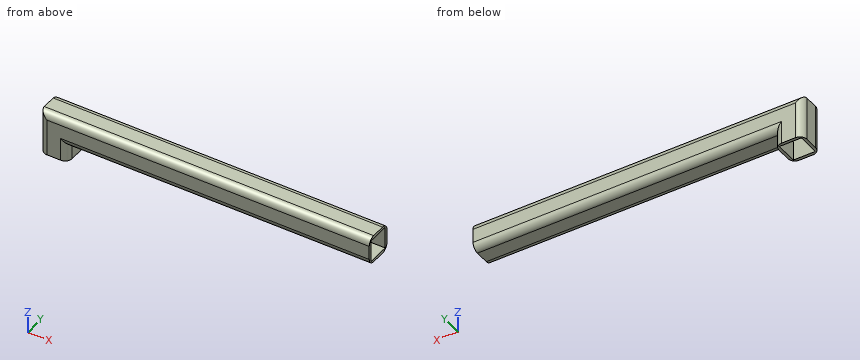
from build123d import *

# Parameters (mm, degrees)
SKETCH12_W = 120.65
SKETCH12_H = 120.65


with BuildPart() as part:
    # Sweep1: sweep along a curve in space
    with BuildLine() as sweep1_path:
        Line((60.325, 60.325, 0), (60.325, 60.325, 165.1))
        Line((60.325, 60.325, 165.1), (1787.525, 60.325, 165.1))
    # Sketch12 → Sweep1 (sweep)
    with BuildSketch(Plane.XY):
        with BuildLine():
            Line((22.225, 136.525), (98.425, 136.525))
            ThreePointArc((98.425, 136.525), (125.365768363, 125.365768363), (136.525, 98.425))
            Line((136.525, 98.425), (136.525, 22.225))
            ThreePointArc((136.525, 22.225), (125.365768363, -4.715768363), (98.425, -15.875))
            Line((98.425, -15.875), (22.225, -15.875))
            ThreePointArc((22.225, -15.875), (-4.715768363, -4.715768363), (-15.875, 22.225))
            Line((-15.875, 22.225), (-15.875, 98.425))
            ThreePointArc((-15.875, 98.425), (-4.715768363, 125.365768363), (22.225, 136.525))
        make_face()
        with Locations((60.325, 60.325)):
            Rectangle(SKETCH12_W, SKETCH12_H, mode=Mode.SUBTRACT)
    sweep(path=sweep1_path.line, transition=Transition.RIGHT)


solid = part.part
Design review of the part built by this model. Coordinates are the model's own, in mm. Give positions to 0.01 mm unless a question says otherwise; leave off trailing zeros. Order: outer loops, then holes, each group sorted by start corner. A loop starts at its lowest first (then second) coordinate and runs counter-clockwise, first axis right, second up.
1. Add section C-C, the plane x = 1498.5. State the section outline as (y, z) points (3 decimals).
Solution:
outline: (-15.875, 127) arc R38.1 ccw to (22.225, 88.9) - (98.425, 88.9) arc R38.1 ccw to (136.525, 127) - (136.525, 203.2) arc R38.1 ccw to (98.425, 241.3) - (22.225, 241.3) arc R38.1 ccw to (-15.875, 203.2) - close; hole (0, 104.775) - (120.65, 104.775) - (120.65, 225.425) - (0, 225.425) - close
2. Add section A-A, the plane y = 50. State the section outline as (x, z) points (3 decimals), then the cut area to 3 significant figures.
Solution:
outline: (-15.875, 0) - (0, 0) - (0, 225.425) - (1787.525, 225.425) - (1787.525, 241.3) - (-15.875, 241.3) - close; (120.65, 0) - (136.525, 0) - (136.525, 88.9) - (1787.525, 88.9) - (1787.525, 104.775) - (120.65, 104.775) - close
area: 60,100 mm2
3. Add section B-B, the plane z = 147.5. State the section outline as (x, y) points (3 decimals).
Solution:
outline: (-15.875, 22.225) arc R38.1 ccw to (22.225, -15.875) - (1787.525, -15.875) - (1787.525, 0) - (0, 0) - (0, 120.65) - (1787.525, 120.65) - (1787.525, 136.525) - (22.225, 136.525) arc R38.1 ccw to (-15.875, 98.425) - close
4. For pin 1 Ø10 at (y, z) = (53, 138.5) entering from +X; pin 2 Ø23 at (x, y) = (666.5, 78) entering from -Z; pin 3 Ø23 at (y, z) = (53, 30) entering from +X (3 decimals), all flat-tipped, find the tip position at first contact; note any pin that passes through.
Solution:
pin 1: stops at x = 0
pin 2: stops at z = 88.9
pin 3: stops at x = 136.525
5. To check wall thickness, follow L1, parallel to Z at x = 611, y = 99 (3 decimals); L2, parallel to Z at x = 730, y = 19.5 (3 decimals); L3, parallel to Y at x = 59, z = 176 (3 decimals). State the ranges of each line that lie inside material, in increasing order.
Solution:
L1: z = 88.904 to 104.775, 225.425 to 241.296
L2: z = 88.998 to 104.775, 225.425 to 241.202
L3: y = -15.875 to 0, 120.65 to 136.525
6. Add section D-D, the plane z = 66.5. State the section outline as (x, y) points (3 decimals), then the cut area to 3 significant figures.
Solution:
outline: (-15.875, 22.225) arc R38.1 ccw to (22.225, -15.875) - (98.425, -15.875) arc R38.1 ccw to (136.525, 22.225) - (136.525, 98.425) arc R38.1 ccw to (98.425, 136.525) - (22.225, 136.525) arc R38.1 ccw to (-15.875, 98.425) - close; hole (0, 0) - (120.65, 0) - (120.65, 120.65) - (0, 120.65) - close
area: 7,420 mm2
